from build123d import *

# Parameters (mm, degrees)
F0_R     = 3.3
F2_R     = 2.3
F4_R     = 1.8
F5_DEPTH = 41.0010001
F6_R     = 6.5
F7_DEPTH = 0.3


with BuildPart() as f3:
    # F0 (on Top) → F3 section 0
    with BuildSketch(Plane.XY):
        Circle(F0_R)
    # F2 (on offset) → F3 section 1
    with BuildSketch(Plane.XY.offset(41)):
        Circle(F2_R)
    loft()

    # F4 (on face) → F5 (cut, through all)
    with BuildSketch(Plane.XY.offset(41)):
        Circle(F4_R)
    extrude(amount=-F5_DEPTH, mode=Mode.SUBTRACT)

    # F6 (on face) → F7 (join)
    with BuildSketch(Plane(origin=(0, 0, 0), x_dir=(1, 0, 0), z_dir=(0, 0, -1))):
        Circle(F6_R)
    extrude(amount=-F7_DEPTH)


solid = f3.part
Part model, mm, in its own coordinate system. A direction names the side the tool comes from. Round coordinates to 2 decimals unless told otherwise and drop trailing zeros. Loops run counter-clockwise (first coordinate to the right, second up) from the corner with the lowest first, then second, coordinate; pieces in that order, holes last. Notation, with made-up numbers: (80, -11.75) - (108, -11.75) arc R27 ccw to (108, 7.25) - close; hole circle Ø7 at (51.5, 65). An arc over 180 degrees is marked (long way). Answer as a JSON object with one key per item and string values.
Item 1: Tool access for faces 1 (the face through (0, -2, 41)), 2 (the face through (1.717, 0.541, 20.935)): list every direction of +Z, -Z, +X, -X, +Y, -Y with a clear straight run to the whole face (end or side of a thin tool).
Output:
{"face 1": "+Z, +X, -X, +Y, -Y", "face 2": "+Z"}
Item 2: Band-saw the part on D-D on z = 37.5. List the corners of the cut face in (x, y).
Output:
{"outline": "circle Ø4.77 at (0, 0); hole circle Ø3.6 at (0, 0)"}
Item 3: Pull direction Y, two halves, no side cores. Call faces 3 (the face through (0, 0, 0.3)), 4 (the face through (-0.605, -2.723, 20.935)), 5 (the face through (-3, -2, 0.3)): pulls with the +Y half, pulls with the -Y half, needs draft (parallel to the pull), parting line crosses it, or undercut.
Output:
{"face 3": "undercut", "face 4": "parting line crosses it", "face 5": "needs draft"}
Item 4: Band-saw the part on B-B on z = 9.5. List the corners of the cut face in (x, y).
Output:
{"outline": "circle Ø6.14 at (0, 0); hole circle Ø3.6 at (0, 0)"}
Item 5: Band-saw the part on A-A on x = 0. List the corners of the cut face in (y, z), plus the area to 3 significant figures.
Output:
{"outline": "(-6.5, 0) - (6.5, 0) - (6.5, 0.3) - (3.29, 0.3) - (2.3, 41) - (1.8, 41) - (1.8, 0.3) - (-1.8, 0.3) - (-1.8, 41) - (-2.3, 41) - (-3.29, 0.3) - (-6.5, 0.3) - close", "area": "85.0 mm2"}
Item 6: Pin check, flat tips, straight feed: pin 1 (6 mm diameter, centred on x = -0.5, z = 4.5, fed in from -Y); pin 2 (1.5 mm diameter, centred on x = -5, z = 6.5, fed in from +Y); pin 3 (4 mm diameter, centred on x = 1, z = 16, fed in from +Y). Stop position of each tip, or through.
Output:
{"pin 1": "y = -3.26", "pin 2": "through", "pin 3": "y = 2.95"}
Item 7: Band-saw the part on C-C on y = -3.75. List the corners of the cut face in (x, z), plus the area to 3 significant figures.
Output:
{"outline": "(-5.31, 0) - (5.31, 0) - (5.31, 0.3) - (-5.31, 0.3) - close", "area": "3.19 mm2"}
Item 8: Wall check: L1, parallel to Y at x = -0.5, z = 29; L2, parallel to Z at x = -0.75, y = -3.5; L3, parallel to X at y = 0.5, z = 4. Give the ranges that are in metal, low to high.
Output:
{"L1": "-2.54 to -1.73, 1.73 to 2.54", "L2": "0 to 0.3", "L3": "-3.16 to -1.73, 1.73 to 3.16"}
